```python
from build123d import *

# Parameters (mm, degrees)
SKETCH1_R           = 16
SKETCH1_R_2         = 2
SKETCH1_R_3         = 3.5
BOSS_EXTRUDE1_DEPTH = 2.5
SKETCH2_R           = 9
SKETCH2_R_2         = 5
CUT_EXTRUDE1_DEPTH  = 1
CHAMFER1_SIZE       = 1


with BuildPart() as part:
    # Sketch1 → Boss-Extrude1 (new body)
    with BuildSketch(Plane.XY):
        Circle(SKETCH1_R)
        with Locations((0, 11.315)):
            Circle(SKETCH1_R_2, mode=Mode.SUBTRACT)
        with Locations((8.000913229, 8.000913229)):
            Circle(SKETCH1_R_2, mode=Mode.SUBTRACT)
        with Locations((11.315, 0)):
            Circle(SKETCH1_R_2, mode=Mode.SUBTRACT)
        with Locations((8.000913229, -8.000913229)):
            Circle(SKETCH1_R_2, mode=Mode.SUBTRACT)
        with Locations((0, -11.315)):
            Circle(SKETCH1_R_2, mode=Mode.SUBTRACT)
        with Locations((-8.000913229, -8.000913229)):
            Circle(SKETCH1_R_2, mode=Mode.SUBTRACT)
        with Locations((-11.315, 0)):
            Circle(SKETCH1_R_2, mode=Mode.SUBTRACT)
        with Locations((-8.000913229, 8.000913229)):
            Circle(SKETCH1_R_2, mode=Mode.SUBTRACT)
        Circle(SKETCH1_R_3, mode=Mode.SUBTRACT)
    extrude(amount=BOSS_EXTRUDE1_DEPTH)

    # Sketch2 → Cut-Extrude1 (cut)
    with BuildSketch(Plane.XY.offset(2.5)):
        Circle(SKETCH2_R)
        Circle(SKETCH2_R_2, mode=Mode.SUBTRACT)
    extrude(amount=-CUT_EXTRUDE1_DEPTH, mode=Mode.SUBTRACT)

    # Chamfer1
    chamfer1_edges = [part.edges().sort_by_distance(p)[0] for p in [
        (-16, 0, 2.5),
    ]]
    chamfer(chamfer1_edges, length=CHAMFER1_SIZE)


solid = part.part
```
The model under review builds one solid part; all positions refer to its coordinate system, in mm. A direction names the side the tool comes from. Give positions to 0.01 mm unless a question says otherwise; leave off trailing zeros. Write each loop counter-clockwise with the first axis right and the second up, starting at its lowest first coordinate (ties: lowest second). Pieces come first, ordered by that corner, then holes.
(1) Consider section C-C, the plane z = 2. Give the number of separate pieces and of enclosed holes in the cut face, and give its area (3 significant figures).
(2) Tool access review of faces 1 (the cylindrical face through (-0.26, -9.33, 1.23)), 2 (the cylindrical face through (-1.172, 8.923, 2.007)): name each direction out of +Z, -Z, +X, -X, +Y, -Y from which nothing blocks a thin tool from reaching the whole face with its end or side.
(3) For P1, Ø6.5, axis at x = -8, y = 8, coming from the +Z side; P2, Ø1, axis at y = -6, z = 2, coming from the +X side, all flat-tipped, find the tip position at first contact; note any pin that passes through.
(4) Consider section A-A, the plane x = 0. Give the boundary of the cut face in (y, z) (3 decimals).
(5) The part is to be moulded in two halves that separate along X. For faces 3 (the flat face through (0, 4, 0)), 4 (the cylindrical face through (-3.47, -15.62, 0.74)), 5 (the cylindrical face through (-7.078, -9.775, 1.232)), say which applies: released by +X, released by -X, zero draft, split by the parting line, or undercut.
(6) To check wall thickness, follow L1, parallel to X at y = 0.5, z = 2; L2, parallel to X at y = 1, z = 1.65; L3, parallel to Y at x = 9, z = 1.05. State the ranges of each line that lie inside material, in increasing order.
Returned:
1. separate pieces: 2
1. enclosed holes: 10
1. area: 440 mm2
2. face 1: +Z, -Z
2. face 2: +Z
3. P1: stops at z = 2.5
3. P2: stops at x = 14.87
4. outline: (-16, 0) - (-13.315, 0) - (-13.315, 2.5) - (-15, 2.5) - (-16, 1.5) - close; (-9.315, 0) - (-3.5, 0) - (-3.5, 2.5) - (-5, 2.5) - (-5, 1.5) - (-9, 1.5) - (-9, 2.5) - (-9.315, 2.5) - close; (3.5, 0) - (9.315, 0) - (9.315, 2.5) - (9, 2.5) - (9, 1.5) - (5, 1.5) - (5, 2.5) - (3.5, 2.5) - close; (13.315, 0) - (16, 0) - (16, 1.5) - (15, 2.5) - (13.315, 2.5) - close
5. face 3: zero draft
5. face 4: split by the parting line
5. face 5: undercut
6. L1: x = -15.49 to -13.25, -9.38 to -8.99, -4.97 to -3.46, 3.46 to 4.97, 8.99 to 9.38, 13.25 to 15.49
6. L2: x = -15.82 to -13.05, -9.58 to -8.94, -4.9 to -3.35, 3.35 to 4.9, 8.94 to 9.58, 13.05 to 15.82
6. L3: y = -13.23 to -9.73, -6.27 to 6.27, 9.73 to 13.23
